```python
from build123d import *

# Parameters (mm, degrees)
SKETCH_1_R                           = 10
EXTRUDE_1_DEPTH                      = 350
FILLET_1_R                           = 1
CUT_EXTRUDE_6_DEPTH                  = 351.285597766
CUT_EXTRUDE_6_DIRECTION_2_REACH      = 352.286
CUT_EXTRUDE_6_DIRECTION_2_END_RADIUS = 9
CUT_EXTRUDE_7_DEPTH                  = 351.285597868
CUT_EXTRUDE_7_DEPTH_BACK             = 351.285597868
SKETCH_7_W                           = 8.4
SKETCH_7_H                           = 16
CUT_EXTRUDE_START                    = -0.924758876
CUT_EXTRUDE_8_DEPTH                  = 11.924758876
CUT_EXTRUDE_START_2                  = 325
CUT_EXTRUDE_8_2_DEPTH                = 7
CUT_EXTRUDE_9_DEPTH                  = 351.285597868
CUT_EXTRUDE_9_DEPTH_BACK             = 351.285597868
SKETCH_9_R                           = 2


with BuildPart() as part:
    # 草图1 → 凸台-拉伸1 (new body)
    with BuildSketch(Plane(origin=(0, 0, 0), x_dir=(1, 0, 0), z_dir=(0, 1, 0))):
        with Locations(Location((0, 0, 0), (0, 0, 270))):
            Circle(SKETCH_1_R)
    extrude(amount=EXTRUDE_1_DEPTH)

    # 圆角1
    fillet_1_edges = [part.edges().sort_by_distance(p)[0] for p in [
        (0, 350, -10),
    ]]
    fillet(fillet_1_edges, radius=FILLET_1_R)

    # 草图5 → 切除-拉伸6 (cut)
    with BuildSketch(Plane.XY):
        with BuildLine():
            Line((3.2, 334), (-3.2, 334))
            ThreePointArc((-3.2, 334), (-3.907106781, 334.292893219), (-4.2, 335))
            Line((-4.2, 335), (-4.2, 366))
            Line((-4.2, 366), (4.2, 366))
            Line((4.2, 366), (4.2, 335))
            ThreePointArc((4.2, 335), (3.907106781, 334.292893219), (3.2, 334))
        make_face()
    extrude(amount=-CUT_EXTRUDE_6_DEPTH, mode=Mode.SUBTRACT)

    # 切除-拉伸6 direction 2: up to this cylinder (the profile starts inside it)
    cut_extrude_6_direction_2_end = Plane(origin=(0, 350.025231, 0), z_dir=(0, -1, 0)) * Cylinder(CUT_EXTRUDE_6_DIRECTION_2_END_RADIUS, 723.572, mode=Mode.PRIVATE)
    # 草图5 → 切除-拉伸6 direction 2 (cut, up to the surface)
    with BuildSketch(Plane.XY, mode=Mode.PRIVATE) as cut_extrude_6_direction_2_sk1:
        with BuildLine():
            Line((3.2, 334), (-3.2, 334))
            ThreePointArc((-3.2, 334), (-3.907106781, 334.292893219), (-4.2, 335))
            Line((-4.2, 335), (-4.2, 366))
            Line((-4.2, 366), (4.2, 366))
            Line((4.2, 366), (4.2, 335))
            ThreePointArc((4.2, 335), (3.907106781, 334.292893219), (3.2, 334))
        make_face()
    cut_extrude_6_direction_2_tool1 = extrude(cut_extrude_6_direction_2_sk1.sketch, amount=CUT_EXTRUDE_6_DIRECTION_2_REACH, mode=Mode.PRIVATE) & cut_extrude_6_direction_2_end
    add(cut_extrude_6_direction_2_tool1.solids().sort_by_distance((0, 350.025231, 0))[0], mode=Mode.SUBTRACT)

    # 草图7 → 切除-拉伸7 (cut, two sides: drawn at the far end of the back side and taken through both)
    with BuildSketch(Plane.XY.offset(-CUT_EXTRUDE_7_DEPTH_BACK)):
        with Locations((0, 350)):
            Rectangle(SKETCH_7_W, SKETCH_7_H)
    extrude(amount=CUT_EXTRUDE_7_DEPTH + CUT_EXTRUDE_7_DEPTH_BACK, mode=Mode.SUBTRACT)

    # 切除-拉伸8: read off the stored shape, not the designer's step
    # 切除-拉伸8 outline → 切除-拉伸8 (cut)
    with BuildSketch(Plane.XY.offset(CUT_EXTRUDE_START)):
        with BuildLine():
            Line((1.7, 331.484532172), (-1.7, 331.484532172))
            add(Edge.make_bspline(
                [(-1.7, 331.484532172), (-2.36531519, 331.484532172), (-2.999142714, 331.215697613), (-3.916295952, 330.308882303), (-4.198882198, 329.654063239), (-4.20111079, 328.323374921), (-3.920415307, 327.665006461), (-2.997944529, 326.751432928), (-2.365478889, 326.484532172), (-1.7, 326.484532172)],
                knots=[0, 0, 0, 0, 0.25, 0.25, 0.5, 0.5, 0.75, 0.75, 1, 1, 1, 1], degree=3))
            Line((-1.7, 326.484532172), (1.7, 326.484532172))
            add(Edge.make_bspline(
                [(1.7, 326.484532172), (2.36531519, 326.484532172), (2.999142714, 326.75336673), (3.916295952, 327.66018204), (4.198882198, 328.315001104), (4.20111079, 329.645689422), (3.920415307, 330.304057882), (2.997944529, 331.217631415), (2.365478889, 331.484532172), (1.7, 331.484532172)],
                knots=[0, 0, 0, 0, 0.25, 0.25, 0.5, 0.5, 0.75, 0.75, 1, 1, 1, 1], degree=3))
        make_face()
    extrude(amount=CUT_EXTRUDE_8_DEPTH, mode=Mode.SUBTRACT)

    # Cut-Extrude 8 2 outline → Cut-Extrude 8 2 (add)
    with BuildSketch(Plane(origin=(0, 0, 0), x_dir=(1, 0, 0), z_dir=(0, 1, 0)).offset(CUT_EXTRUDE_START_2)):
        with BuildLine():
            ThreePointArc((-4.199999886, 0.924758903), (0, 0), (4.199999886, 0.924758903))
            Line((4.199999886, 0.924758903), (-4.199999886, 0.924758903))
        make_face()
    extrude(amount=CUT_EXTRUDE_8_2_DEPTH)

    # 草图9 → 切除-拉伸9 (cut, two sides: drawn at the far end of the back side and taken through both)
    with BuildSketch(Plane(origin=(0, 0, 0), x_dir=(0, 0, -1), z_dir=(1, 0, 0)).offset(-CUT_EXTRUDE_9_DEPTH_BACK)):
        with Locations((0, 342.814995951)):
            Circle(SKETCH_9_R)
    extrude(amount=CUT_EXTRUDE_9_DEPTH + CUT_EXTRUDE_9_DEPTH_BACK, mode=Mode.SUBTRACT)


solid = part.part
```
Check sheet for the modelled part. Datum: model origin and axes. Units: mm. Coordinates: 2 decimals unless noted, no trailing zeros. Order: outer loops, then holes, each group sorted by start corner. A loop starts at its lowest first (then second) coordinate and runs counter-clockwise, first axis right, second up. Notation, with made-up numbers: (83.5, 4.25) -> (132.5, 4.25) arc R23 cw to (132.5, 36.25) -> close; hole circle Ø10 at (50, 48). An arc over 180 degrees is marked (long way). Write each question's results on one line, items separated by ' | '. Start each with the question number.
1) Section check A-A (y = 188). Enter the section's corners in (x, z), and give its area (3 significant figures).
2) Depth check by flat-ended pin: pin 1 (1.9 mm diameter, centred on x = 0, z = 3.5, fed in from +Y); pin 2 (0.6 mm diameter, centred on x = -2, z = 9.5, fed in from +Y); pin 3 (2 mm diameter, centred on y = 47, z = -5, fed in from +X); pin 4 (3 mm diameter, centred on y = 342.81, z = 0, fed in from +X). Enter the tip coordinate at first touch or a pass-through.
3) Material ranges on line 1 along Y through (x, z) = (-1, 5.5); line 2 along Y through (x, z) = (6.6, 0) (3 decimals); line 3 along Y through (x, z) = (-3.5, -1.5), recorded low to high.
4) Draft check along X on faces 1 (the face through (0, 0, 0)), 2 (the face through (-6, 172, -8)), 3 (the face through (0, 334, 0)). Enter one of: pulls with the +X half, pulls with the -X half, needs draft (parallel to the pull), parting line crosses it, or undercut.
Checked values:
1) outline: circle Ø20 at (0, 0) | area: 314 mm²
2) pin 1: y = 334 | pin 2: y = 342 | pin 3: x = 9.17 | pin 4: through
3) line 1: 0 to 326.48, 331.48 to 334 | line 2: 0 to 340.815, 344.815 to 350 | line 3: 0 to 334.05
4) face 1: needs draft | face 2: parting line crosses it | face 3: undercut
